Work out the finished part from the listing and answer in its coordinate system (mm). A direction names the side the tool comes from. Give positions to 0.01 mm unless a question says otherwise; leave off trailing zeros. Loops run counter-clockwise (first coordinate to the right, second up) from the corner with the lowest first, then second, coordinate; pieces in that order, holes last. Notation, with made-up numbers: (-26, 30.5) - (-7, 30.5) arc R13 ccw to (-7, 43.5) - close; hole circle Ø5 at (44.25, 7). An arc over 180 degrees is marked (long way). Use CSV: the item, a comma, the result in double quotes.
from build123d import *

# Parameters (mm, degrees)
EXTRUDE_2_DEPTH     = 5
SKETCH_4_W          = 33
SKETCH_4_H          = 4
EXTRUDE_3_DEPTH     = 23
EXTRUDE_4_DEPTH     = 33
SKETCH_11_R         = 2
CUT_EXTRUDE_1_DEPTH = 14
CUT_EXTRUDE_2_DEPTH = 33
SKETCH_17_R         = 2
CUT_EXTRUDE_3_DEPTH = 5
SKETCH_18_W         = 37
SKETCH_18_H         = 3
EXTRUDE_5_DEPTH     = 5
SKETCH_19_W         = 55
SKETCH_19_H         = 4.170749575
EXTRUDE_6_DEPTH     = 5
SKETCH_21_R         = 2
CUT_EXTRUDE_4_DEPTH = 5
FILLET_1_R          = 1
EXTRUDE_10_DEPTH    = 33


with BuildPart() as part:
    # 草图1 → 凸台-拉伸2 (new body)
    with BuildSketch(Plane(origin=(0, 0, 0), x_dir=(1, 0, 0), z_dir=(0, 1, 0))):
        with BuildLine():
            Line((26.533821687, -5), (18.533821687, -5))
            ThreePointArc((18.533821687, -5), (17.826714906, -4.707106781), (17.533821687, -4))
            Line((17.533821687, -4), (17.533821687, -3))
            ThreePointArc((17.533821687, -3), (17.240928468, -2.292893219), (16.533821687, -2))
            Line((16.533821687, -2), (-16.466178313, -2))
            ThreePointArc((-16.466178313, -2), (-17.173285094, -2.292893219), (-17.466178313, -3))
            Line((-17.466178313, -3), (-17.466178313, -4))
            ThreePointArc((-17.466178313, -4), (-17.759071532, -4.707106781), (-18.466178313, -5))
            Line((-18.466178313, -5), (-26.466178313, -5))
            ThreePointArc((-26.466178313, -5), (-27.173285094, -4.707106781), (-27.466178313, -4))
            Line((-27.466178313, -4), (-27.466178313, 4))
            ThreePointArc((-27.466178313, 4), (-27.173285094, 4.707106781), (-26.466178313, 5))
            Line((-26.466178313, 5), (-18.466178313, 5))
            ThreePointArc((-18.466178313, 5), (-17.759071532, 4.707106781), (-17.466178313, 4))
            Line((-17.466178313, 4), (-17.466178313, 3))
            ThreePointArc((-17.466178313, 3), (-17.173285094, 2.292893219), (-16.466178313, 2))
            Line((-16.466178313, 2), (16.533821687, 2))
            ThreePointArc((16.533821687, 2), (17.240928468, 2.292893219), (17.533821687, 3))
            Line((17.533821687, 3), (17.533821687, 4))
            ThreePointArc((17.533821687, 4), (17.826714906, 4.707106781), (18.533821687, 5))
            Line((18.533821687, 5), (26.533821687, 5))
            ThreePointArc((26.533821687, 5), (27.240928468, 4.707106781), (27.533821687, 4))
            Line((27.533821687, 4), (27.533821687, -4))
            ThreePointArc((27.533821687, -4), (27.240928468, -4.707106781), (26.533821687, -5))
        make_face()
    extrude(amount=EXTRUDE_2_DEPTH)

    # 草图4 → 凸台-拉伸3 (add)
    with BuildSketch(Plane(origin=(0, 5, 0), x_dir=(1, 0, 0), z_dir=(0, 1, 0))):
        with Locations((0.033821687, 0)):
            Rectangle(SKETCH_4_W, SKETCH_4_H)
    extrude(amount=EXTRUDE_3_DEPTH)

    # 草图5 → 凸台-拉伸4 (add)
    with BuildSketch(Plane.ZY.offset(16.466178313)):
        with BuildLine():
            ThreePointArc((2, 27.585786438), (2.076120467, 27.96846987), (2.292893219, 28.292893219))
            Line((2.292893219, 28.292893219), (19.970562748, 45.970562748))
            Line((19.970562748, 45.970562748), (17.970562748, 47.970562748))
            Line((17.970562748, 47.970562748), (-1.707106781, 28.292893219))
            ThreePointArc((-1.707106781, 28.292893219), (-1.821797126, 28.155566643), (-1.910179721, 28))
            Line((-1.910179721, 28), (2, 28))
            Line((2, 28), (2, 27.585786438))
        make_face()
    extrude(amount=-EXTRUDE_4_DEPTH)

    # 草图11 → 切除-拉伸1 (cut)
    with BuildSketch(Plane.XY.offset(2)):
        with Locations((13.533821687, 22.143107046)):
            Circle(SKETCH_11_R)
        with Locations((13.533821687, 13.028465829)):
            Circle(SKETCH_11_R)
        with BuildLine():
            Line((-11.034001398, 22.143107046), (-11.034001398, 13.028465829))
            ThreePointArc((-11.034001398, 13.028465829), (-12.750089855, 11.312377371), (-14.466178313, 13.028465829))
            Line((-14.466178313, 13.028465829), (-14.466178313, 22.143107046))
            ThreePointArc((-14.466178313, 22.143107046), (-12.750089855, 23.859195504), (-11.034001398, 22.143107046))
        make_face()
    extrude(amount=-CUT_EXTRUDE_1_DEPTH, mode=Mode.SUBTRACT)

    # 草图16 → 切除-拉伸2 (cut)
    with BuildSketch(Plane.ZY.offset(16.466178313)):
        with BuildLine():
            Line((-1.910179721, 28), (-2, 28))
            Line((-2, 28), (-2, 27.585786438))
            ThreePointArc((-2, 27.585786438), (-1.97728699, 27.797706563), (-1.910179721, 28))
        make_face()
    extrude(amount=-CUT_EXTRUDE_2_DEPTH, mode=Mode.SUBTRACT)

    # 草图17 → 切除-拉伸3 (cut)
    with BuildSketch(Plane(origin=(0, 5, 0), x_dir=(1, 0, 0), z_dir=(0, 1, 0))):
        with Locations((22.533821687, 0)):
            Circle(SKETCH_17_R)
        with Locations((-22.466178313, 0)):
            Circle(SKETCH_17_R)
    extrude(amount=-CUT_EXTRUDE_3_DEPTH, mode=Mode.SUBTRACT)

    # 草图18 → 凸台-拉伸5 (add)
    with BuildSketch(Plane.XZ):
        with Locations((0.033821687, -3.5)):
            Rectangle(SKETCH_18_W, SKETCH_18_H)
    extrude(amount=-EXTRUDE_5_DEPTH)

    # 草图19 → 凸台-拉伸6 (add)
    with BuildSketch(Plane.XZ):
        with Locations((0.033821687, -4.914625212)):
            Rectangle(SKETCH_19_W, SKETCH_19_H)
    extrude(amount=-EXTRUDE_6_DEPTH)

    # 草图21 → 切除-拉伸4 (cut)
    with BuildSketch(Plane.XZ):
        with Locations((-16.966178313, -4.5)):
            Circle(SKETCH_21_R)
        with Locations((16.966178313, -4.5)):
            Circle(SKETCH_21_R)
    extrude(amount=-CUT_EXTRUDE_4_DEPTH, mode=Mode.SUBTRACT)

    # 圆角1
    fillet_1_edges = [part.edges().sort_by_distance(p)[0] for p in [
        (27.533821687, 2.5, -7),
        (-27.466178313, 2.5, -7),
    ]]
    fillet(fillet_1_edges, radius=FILLET_1_R)

    # 草图29 → 凸台-拉伸10 (add)
    with BuildSketch(Plane(origin=(16.533821687, 0, 0), x_dir=(0, 0, -1), z_dir=(1, 0, 0))):
        with BuildLine():
            Line((-2, 5.537377417), (-2, 5))
            ThreePointArc((-2, 5), (-19.470562748, 21.763455967), (-19.970562748, 45.970562748))
            Line((-19.970562748, 45.970562748), (-19.583896385, 45.583896385))
            ThreePointArc((-19.583896385, 45.583896385), (-19.007789844, 21.953169584), (-2, 5.537377417))
        make_face()
    extrude(amount=-EXTRUDE_10_DEPTH)


solid = part.part
Item 1: The mould has two halves that part along Z. Classify faces 6 (the flat face through (27.534, 2, -1)), 7 (the flat face through (-0.2, 46.96, 18.98)), 8 (the flat face through (0, 16, 2)): pulls with the +Z half, pulls with the -Z half, needs draft (parallel to the pull), parting line crosses it, or undercut.
Determined:
face 6,"needs draft"
face 7,"pulls with the +Z half"
face 8,"undercut"
Item 2: Find the intervals of material crossed by line 1 (X direction, y = 2.6, z = 0); line 2 (X direction, y = 13.5, z = 1); line 3 (Z direction, x = -19, y = 4), in increasing order.
Determined:
line 1,"x = -27.47 to -24.47, -20.47 to 20.53, 24.53 to 27.53"
line 2,"x = -16.47 to -14.47, -11.03 to 11.59, 15.48 to 16.53"
line 3,"z = -7 to 5"
Item 3: A cutting plane is placed at C-C on y = 16.5. Determine the outline of the cut face in (x, z), and give its area (3 significant figures).
Determined:
outline,"(-16.47, -2) - (-14.47, -2) - (-14.47, 2) - (-16.47, 2) - close; (-16.47, 15.93) - (16.53, 15.93) - (16.53, 16.54) - (-16.47, 16.54) - close; (-11.03, -2) - (16.53, -2) - (16.53, 2) - (-11.03, 2) - close"
area,"138 mm²"
Item 4: For faces 1 (the flat face through (0, 2, -7)), 2 (the flat face through (16.534, 23, 1)), 3 (the flat face through (0, 16, -2)), 4 (the cylindrical face through (15.38, 2.46, -5.72)), 5 (the cylindrical face through (-12.79, 23.86, 0.03)), determine the directions among +Z, -Z, +X, -X, +Y, -Y from which every point of the face is accessible in a straight line to the end or side of a thin tool.
Determined:
face 1,"-Z, +X, -X, +Y, -Y"
face 2,"+Z, -Z, +X, +Y"
face 3,"-Z, +X, -X, +Y"
face 4,"+Y, -Y"
face 5,"-Z"
Item 5: A cutting plane is placed at D-D on x = -9. Determine the outline of the cut face in (y, z).
Determined:
outline,"(0, -7) - (5, -7) - (5, -2) - (27.59, -2) arc R1 ccw to (28.29, -1.71) - (47.97, 17.97) - (45.97, 19.97) arc R31.63 ccw to (5, 2) - (0, 2) - close; hole (5.54, 2) - (27.59, 2) arc R1 ccw to (28.29, 2.29) - (45.58, 19.58) arc R31.13 ccw to start"
Item 6: A cutting plane is placed at B-B on z = -4.5. Determine the outline of the cut face in (x, y).
Determined:
outline,"(-27.47, 0) - (-18.97, 0) - (-18.97, 5) - (-27.47, 5) - close; (-14.97, 0) - (14.97, 0) - (14.97, 5) - (-14.97, 5) - close; (18.97, 0) - (27.53, 0) - (27.53, 5) - (18.97, 5) - close"
Item 7: A cutting plane is placed at A-A on z = 0. Determine the outline of the cut face in (x, y).
Determined:
outline,"(-27.47, 0) - (-24.47, 0) - (-24.47, 5) - (-27.47, 5) - close; (-20.47, 0) - (20.53, 0) - (20.53, 5) - (16.53, 5) - (16.53, 30) - (-16.47, 30) - (-16.47, 5) - (-20.47, 5) - close; (24.53, 0) - (27.53, 0) - (27.53, 5) - (24.53, 5) - close; hole (-14.47, 13.03) arc R1.72 ccw to (-11.03, 13.03) - (-11.03, 22.14) arc R1.72 ccw to (-14.47, 22.14) - close; hole circle Ø4 at (13.53, 13.03); hole circle Ø4 at (13.53, 22.14)"
Item 8: Given P1, Ø24.5, axis at x = -4, y = 18, coming from the +Z side; P2, Ø4, axis at x = -5, y = 2.5, coming from the +Z side; P3, Ø6, axis at x = -20, z = -2.5, coming from the -Y side; P4, Ø4.5, axis at y = 17, z = 1, coming from the +X side, each flat-ended and moving along its own axis, determine where each tip first touches the part or whether it passes through.
Determined:
P1,"stops at z = 21.85"
P2,"stops at z = 2"
P3,"stops at y = 0"
P4,"stops at x = 16.53"
